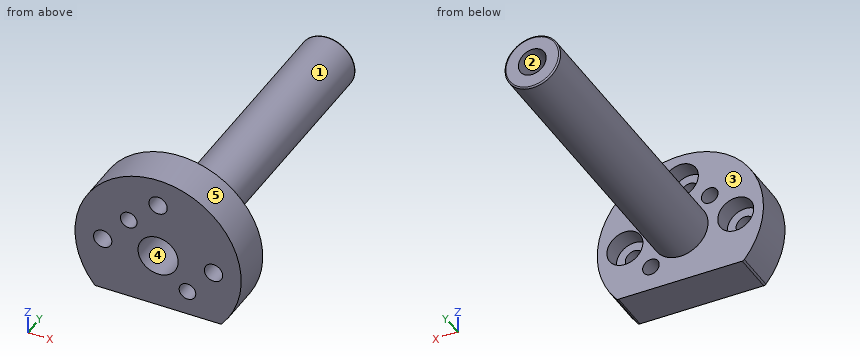
```python
from build123d import *

# Parameters (mm, degrees)
BOSS_EXTRUDE1_DEPTH = 15
SKETCH2_R           = 10
BOSS_EXTRUDE2_DEPTH = 103
SKETCH4_R           = 7.25
CUT_EXTRUDE1_DEPTH  = 57
SKETCH5_R           = 5
CUT_EXTRUDE2_DEPTH  = 62
SKETCH7_R           = 6.5
CUT_EXTRUDE3_DEPTH  = 6.6
SKETCH8_R           = 3.3
CUT_EXTRUDE4_DEPTH  = 9.4
CIRPATTERN1_COUNT   = 4
FILLET1_R           = 0.5
FILLET2_R           = 1
SKETCH9_R           = 3
CUT_EXTRUDE5_DEPTH  = 16


with BuildPart() as part:
    # Sketch1 → Boss-Extrude1 (new body)
    with BuildSketch(Plane(origin=(0, 0, 0), x_dir=(1, 0, 0), z_dir=(0, 1, 0))):
        with BuildLine():
            Line((22.79802623, 19.5), (-22.79802623, 19.5))
            ThreePointArc((-22.79802623, 19.5), (0, -30), (22.79802623, 19.5))
        make_face()
    extrude(amount=BOSS_EXTRUDE1_DEPTH)

    # Sketch2 → Boss-Extrude2 (add)
    with BuildSketch(Plane(origin=(0, 15, 0), x_dir=(1, 0, 0), z_dir=(0, 1, 0))):
        Circle(SKETCH2_R)
    extrude(amount=BOSS_EXTRUDE2_DEPTH)

    # Sketch4 → Cut-Extrude1 (cut)
    with BuildSketch(Plane.XZ):
        Circle(SKETCH4_R)
    extrude(amount=-CUT_EXTRUDE1_DEPTH, mode=Mode.SUBTRACT)

    # Sketch5 → Cut-Extrude2 (cut, through all)
    with BuildSketch(Plane.XZ.offset(-57)):
        Circle(SKETCH5_R)
    extrude(amount=-CUT_EXTRUDE2_DEPTH, mode=Mode.SUBTRACT)

    # Sketch7 → Cut-Extrude3 (cut)
    with BuildSketch(Plane(origin=(0, 15, 0), x_dir=(1, 0, 0), z_dir=(0, 1, 0))):
        with Locations((0, -20)):
            Circle(SKETCH7_R)
    cut_extrude3 = extrude(amount=-CUT_EXTRUDE3_DEPTH, mode=Mode.SUBTRACT)

    # Sketch8 → Cut-Extrude4 (cut, through all)
    with BuildSketch(Plane(origin=(0, 8.4, 0), x_dir=(1, 0, 0), z_dir=(0, 1, 0))):
        with Locations((0, -20)):
            Circle(SKETCH8_R)
    cut_extrude4 = extrude(amount=-CUT_EXTRUDE4_DEPTH, mode=Mode.SUBTRACT)

    # CirPattern1: Cut-Extrude3, Cut-Extrude4 ×4 about axis, 1 skipped
    cirpattern1_axis = Axis((0, 0, 0), (0, -1, 0))
    add([cut_extrude3.rotate(cirpattern1_axis, i * 360 / CIRPATTERN1_COUNT) for i in range(1, CIRPATTERN1_COUNT) if i not in (2,)], mode=Mode.SUBTRACT)
    add([cut_extrude4.rotate(cirpattern1_axis, i * 360 / CIRPATTERN1_COUNT) for i in range(1, CIRPATTERN1_COUNT) if i not in (2,)], mode=Mode.SUBTRACT)

    # Fillet1
    fillet1_edges = [part.edges().sort_by_distance(p)[0] for p in [
        (-10, 118, 0),
    ]]
    fillet(fillet1_edges, radius=FILLET1_R)

    # Fillet2
    fillet2_edges = [part.edges().sort_by_distance(p)[0] for p in [
        (-22.79802623, 7.5, -19.5),
        (22.79802623, 7.5, -19.5),
    ]]
    fillet(fillet2_edges, radius=FILLET2_R)

    # Sketch9 → Cut-Extrude5 (cut, through all)
    with BuildSketch(Plane(origin=(0, 15, 0), x_dir=(1, 0, 0), z_dir=(0, 1, 0))):
        with Locations((-10.606601718, -10.606601718)):
            Circle(SKETCH9_R)
        with Locations((10.606601718, 10.606601718)):
            Circle(SKETCH9_R)
    extrude(amount=-CUT_EXTRUDE5_DEPTH, mode=Mode.SUBTRACT)


solid = part.part
```
The model under review builds one solid part; all positions refer to its coordinate system, in mm. Face numbers are marked on the shaded views. A direction names the side the tool comes from. Give positions to 0.01 mm unless a question says otherwise; leave off trailing zeros. Write each loop counter-clockwise with the first axis right and the second up, starting at its lowest first coordinate (ties: lowest second). Pieces come first, ordered by that corner, then holes. Notation, with made-up numbers: M -26.5,78 L -16.5,78 A35 ccw -16.5,117 Z; hole C 72,-22.5 d3. An arc over 180 degrees is marked long. Answer in a Markdown table with one row per item.
Item 1: Add section D-D on z = 20. Give the boundary of the cut face in (x, y).
Check sheet entries:
| item | result |
|---|---|
| outline | M -22.36,0 L -3.3,0 L -3.3,8.4 L -6.5,8.4 L -6.5,15 L -22.36,15 Z; M 3.3,0 L 22.36,0 L 22.36,15 L 6.5,15 L 6.5,8.4 L 3.3,8.4 Z |
Item 2: Add section A-A on z = 0. State how many separate pieces and enclosed holes the cut face has, plus the area to 3 significant figures.
Check sheet entries:
| item | result |
|---|---|
| separate pieces | 4 |
| enclosed holes | 0 |
| area | 1,240 mm2 |
Item 3: Tool access review of the marked faces 4 and 5: name each direction out of +Z, -Z, +X, -X, +Y, -Y from which nothing blocks a thin tool from reaching the whole face with its end or side.
Check sheet entries:
| item | result |
|---|---|
| face 4 | -Y |
| face 5 | +Y, -Y |
Item 4: Add section C-C on x = 20. Give the boundary of the cut face in (y, z), plus the area to 3 significant figures.
Check sheet entries:
| item | result |
|---|---|
| outline | M 0,-19.5 L 15,-19.5 L 15,-6.5 L 8.4,-6.5 L 8.4,-3.3 L 0,-3.3 Z; M 0,3.3 L 8.4,3.3 L 8.4,6.5 L 15,6.5 L 15,22.36 L 0,22.36 Z |
| area | 487 mm2 |
Item 5: For line 1 along Z through (x, y) = (20, 6.25); line 2 along Z through (x, y) = (0, 6.75); line 3 along X through (y, z) = (12.75, 20), list the stretches that pass through material, from the lowest coordinate up.
Check sheet entries:
| item | result |
|---|---|
| line 1 | -19.5 to -3.3, 3.3 to 22.36 |
| line 2 | -19.5 to -7.25, 7.25 to 16.7, 23.3 to 30 |
| line 3 | -22.36 to -6.5, 6.5 to 22.36 |
Item 6: For P1, Ø9.5, axis at x = -10.61, z = 10.61, coming from the +Y side; P2, Ø13, axis at x = 0, z = 0, coming from the -Y side; P3, Ø1.5, axis at x = 5.5, y = 104, coming from the +Z side, all flat-tipped, find the tip position at first contact; note any pin that passes through.
Check sheet entries:
| item | result |
|---|---|
| P1 | y = 15 |
| P2 | y = 57 |
| P3 | z = 8.8 |
Item 7: Add section B-B on x = 0. Give the boundary of the cut face in (y, z), plus the area to 3 significant figures.
Check sheet entries:
| item | result |
|---|---|
| outline | M 0,-19.5 L 15,-19.5 L 15,-10 L 117.5,-10 A0.5 ccw 118,-9.5 L 118,-5 L 57,-5 L 57,-7.25 L 0,-7.25 Z; M 0,7.25 L 57,7.25 L 57,5 L 118,5 L 118,9.5 A0.5 ccw 117.5,10 L 15,10 L 15,13.5 L 8.4,13.5 L 8.4,16.7 L 0,16.7 Z; M 0,23.3 L 8.4,23.3 L 8.4,26.5 L 15,26.5 L 15,30 L 0,30 Z |
| area | 1,220 mm2 |
Item 8: Draft analysis for pull direction X (two halves, no side actions). For the marked faces 1, 2 and 3, state which applies: +X half, -X half, draft (parallel to the pull), parting line (faces both ways), or undercut.
Check sheet entries:
| item | result |
|---|---|
| face 1 | parting line |
| face 2 | undercut |
| face 3 | draft |
